Source: CAD feature listing. Evaluate the final solid. Frame: model axes, mm. A direction names the side the tool comes from. Round coordinates to 2 decimals unless told otherwise and drop trailing zeros. Write each loop counter-clockwise with the first axis right and the second up, starting at its lowest first coordinate (ties: lowest second). Pieces come first, ordered by that corner, then holes. Notation, with made-up numbers: M -2.75,-15 L 50.25,-15 A18 cw 50.25,-8 Z; hole C 15.25,68.25 d1. An arc over 180 degrees is marked long. Answer in a Markdown table with one row per item. Add a question column.
Item 1: Material intervals for probe 1 along Z at (x, y) = (1.5, 15); probe 2 along Y at (x, z) = (-0.4, -2.3); probe 3 along Z at (x, y) = (2.6, 18.5), sorted ascending.
Item 2: Cut plane D-D on z = -1.4. Return loops of the section in (x, y), and give its area (3 significant figures).
Item 3: Contact query for flat-ended pins moving along their axis: pin 1 (1 mm diameter, centred on x = -1, z = 1.5, fed in from -Y); pin 2 (1 mm diameter, centred on y = 6, z = 1, fed in from +X). Output: stop coordinate, or through.
Item 4: Set-up query: faces 1 (the face through (0, 4.8, -2.5)), 2 (the face through (0, 20, 0)), 3 (the face through (0, 4.8, 2.4)). Return all of +Z, -Z, +X, -X, +Y, -Y with unobstructed straight access to the full face (end or side cutting, diameter ignored); none if empty.
Item 5: Cut plane A-A on x = 0. Return loops of the section in (y, z), and give its area (3 significant figures).
Item 6: Cut plane B-B on y = 3.5. Return loops of the section in (x, z).
Item 7: Cut plane C-C on x = -1.8. Return loops of the section in (y, z).
from build123d import *

# Parameters (mm, degrees)
SKETCH_1_R          = 3
EXTRUDE_1_DEPTH     = 20
CUT_EXTRUDE_START   = -15.2
CUT_EXTRUDE_2_DEPTH = 15.2


with BuildPart() as part:
    # 草图1 → 凸台-拉伸1 (new body)
    with BuildSketch(Plane(origin=(0, 0, 0), x_dir=(1, 0, 0), z_dir=(0, 1, 0))):
        with Locations(Location((0, 0, 0), (0, 0, 270))):
            Circle(SKETCH_1_R)
    extrude(amount=EXTRUDE_1_DEPTH)

    # 草图2 → 切除-拉伸2 (cut)
    with BuildSketch(Plane(origin=(0, 20, 0), x_dir=(1, 0, 0), z_dir=(0, 1, 0)).offset(CUT_EXTRUDE_START)):
        with BuildLine():
            Line((-2.142428529, 2.1), (2.142428529, 2.1))
            ThreePointArc((2.142428529, 2.1), (0, 3), (-2.142428529, 2.1))
        make_face()
        with BuildLine():
            Line((-2.142428529, -2.1), (2.142428529, -2.1))
            ThreePointArc((2.142428529, -2.1), (0, -3), (-2.142428529, -2.1))
        make_face()
    extrude(amount=CUT_EXTRUDE_2_DEPTH, mode=Mode.SUBTRACT)


solid = part.part
Results below:
| question | item | result |
|---|---|---|
| 1 | probe 1 | -2.1 to 2.1 |
| 1 | probe 2 | 0 to 4.8 |
| 1 | probe 3 | -1.5 to 1.5 |
| 2 | outline | M -2.65,0 L 2.65,0 L 2.65,20 L -2.65,20 Z |
| 2 | area | 106 mm2 |
| 3 | pin 1 | y = 0 |
| 3 | pin 2 | x = 2.96 |
| 4 | face 1 | -Z, +X, -X, +Y |
| 4 | face 2 | +Z, -Z, +X, -X, +Y |
| 4 | face 3 | +Z, +X, -X, +Y |
| 5 | outline | M 0,-3 L 4.8,-3 L 4.8,-2.1 L 20,-2.1 L 20,2.1 L 4.8,2.1 L 4.8,3 L 0,3 Z |
| 5 | area | 92.6 mm2 |
| 6 | outline | C 0,0 d6 |
| 7 | outline | M 0,-2.4 L 4.8,-2.4 L 4.8,-2.1 L 20,-2.1 L 20,2.1 L 4.8,2.1 L 4.8,2.4 L 0,2.4 Z |
